```python
from build123d import *

# Parameters (mm, degrees)
F1_DEPTH      = 7.4
F1_DEPTH_BACK = 7.4
F3_W          = 18
F3_H          = 3
F4_DEPTH      = 25
F4_DEPTH_BACK = 25
F2_R          = 2.75
F5_DEPTH      = 25
F5_DEPTH_BACK = 25
F6_R          = 5.5
F7_DEPTH      = 3
F8_R          = 0.5
F9_R          = 1
F10_DEPTH     = 1


with BuildPart() as f1:
    # F0 (on Front) → F1 (new body, two sides)
    with BuildSketch(Plane.XZ) as f1_sk:
        with BuildLine():
            Line((-32.6, -7.4), (32.6, -7.4))
            ThreePointArc((32.6, -7.4), (37.8325901808, -5.2325901808), (40, 0))
            ThreePointArc((40, 0), (37.8325901808, 5.2325901808), (32.6, 7.4))
            Line((32.6, 7.4), (-32.6, 7.4))
            ThreePointArc((-32.6, 7.4), (-37.8325901808, 5.2325901808), (-40, 0))
            ThreePointArc((-40, 0), (-37.8325901808, -5.2325901808), (-32.6, -7.4))
        make_face()
    extrude(amount=F1_DEPTH)
    extrude(f1_sk.sketch, amount=-F1_DEPTH_BACK)

    # F3 (on Top) → F4 (cut, two sides)
    with BuildSketch(Plane.XY) as f4_sk:
        with Locations((-32.5, 6)):
            Rectangle(F3_W, F3_H)
        with Locations((-32.5, 0)):
            Rectangle(F3_W, F3_H)
        with Locations((-32.5, -6)):
            Rectangle(F3_W, F3_H)
        with Locations((32.5, 3)):
            Rectangle(F3_W, F3_H)
        with Locations((32.5, -3)):
            Rectangle(F3_W, F3_H)
    extrude(amount=F4_DEPTH, mode=Mode.SUBTRACT)
    extrude(f4_sk.sketch, amount=-F4_DEPTH_BACK, mode=Mode.SUBTRACT)

    # F2 (on Front) → F5 (cut, two sides)
    with BuildSketch(Plane.XZ) as f5_sk:
        with Locations((-33, 0)):
            Circle(F2_R)
        with Locations((33, 0)):
            Circle(F2_R)
    extrude(amount=-F5_DEPTH, mode=Mode.SUBTRACT)
    extrude(f5_sk.sketch, amount=F5_DEPTH_BACK, mode=Mode.SUBTRACT)

    # F6 (on face) → F7 (join)
    with BuildSketch(Plane.XZ.offset(7.4)):
        with Locations((33, 0)):
            Circle(F6_R)
        Polygon((37.6188021535, 0), (35.3094010768, -4), (30.6905989232, -4), (28.3811978465, 0), (30.6905989232, 4), (35.3094010768, 4), align=None, mode=Mode.SUBTRACT)
    extrude(amount=F7_DEPTH)

    # F8
    f8_edges = [f1.edges().sort_by_distance(p)[0] for p in [
        (27.5, -10.4, 0),
    ]]
    fillet(f8_edges, radius=F8_R)

    # F9
    f9_edges = [f1.edges().sort_by_distance(p)[0] for p in [
        (27.5, -7.4, 0),
    ]]
    fillet(f9_edges, radius=F9_R)

    # F10 (add): a face of the model
    f10_faces = [f1.faces().sort_by_distance(p)[0] for p in [
        (36.3582715627, -7.4, -1.9388989907),
    ]]
    extrude(f10_faces, amount=F10_DEPTH)


solid = f1.part
```
Geometry check sheet. Reference: the model listing, model coordinates, mm. A direction names the side the tool comes from. Coordinates: 2 decimals unless noted, no trailing zeros. Loops run counter-clockwise (first coordinate to the right, second up) from the corner with the lowest first, then second, coordinate; pieces in that order, holes last.
Item 1: Sectioned sample at B-B, the plane x = -14. Record the boundary of the cut face in (y, z).
Item 2: Sectioned sample at A-A, the plane y = -6. Record the boundary of the cut face in (x, z).
Item 3: Release check for a two-part mould opening along X. For faces 5 (the face through (36.48, -9.39, -1.97)), 6 (the face through (23.5, -3, 0)), 7 (the face through (33, -9, 4)), 8 (the face through (30, -4.5, 0)) record: released by +X, released by -X, zero draft, split by the parting line, or undercut.
Item 4: Access from +Z, -Z, +X, -X, +Y, -Y to the whole of each face (thin tool, end or side, straight path). Record for faces 1 (the face through (-23.5, 6, 0)), 2 (the face through (30, 4.5, 0)), 3 (the face through (-23.5, -6, 0)), 4 (the face through (33, -9, -4)).
Item 5: Thickness scan on line 1 (Y direction, x = 25, z = 1.75); line 2 (Z direction, x = -33, y = -2.95); line 3 (Y direction, x = 36, z = 1). Record the ranges inside material, lowest first.
Item 6: Go/stop test with flat-tipped pins: pin 1 Ø1.5 at (y, z) = (5.5, 4) entering from -X; pin 2 Ø2 at (x, z) = (-13, 5.5) entering from -Y; pin 3 Ø7 at (x, z) = (-33, 0) entering from +Y; pin 4 Ø5 at (x, z) = (33, 0) entering from -Y. Record where each tip stops, or that it passes through.
Check result:
1. outline: (-7.4, -7.4) - (7.4, -7.4) - (7.4, 7.4) - (-7.4, 7.4) - close
2. outline: (-23.5, -7.4) - (32.6, -7.4) arc R7.4 ccw to (32.6, 7.4) - (-23.5, 7.4) - close; hole circle Ø5.5 at (33, 0)
3. face 5: undercut
3. face 6: released by +X
3. face 7: undercut
3. face 8: zero draft
4. face 1: +Z, -Z, -X, +Y
4. face 2: +Z, -Z, +X
4. face 3: +Z, -Z, -X, -Y
4. face 4: -Y
5. line 1: y = -7.4 to -4.5, -1.5 to 1.5, 4.5 to 7.4
5. line 2: z = -7.39 to -2.75, 2.75 to 7.39
5. line 3: y = -8.4 to -4.5, -1.5 to 1.5, 4.5 to 7.4
6. pin 1: stops at x = -23.5
6. pin 2: stops at y = -7.4
6. pin 3: stops at y = 4.5
6. pin 4: passes through
